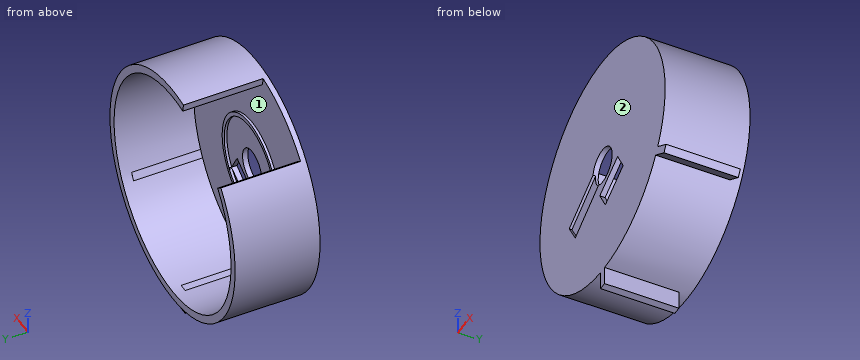
```python
from build123d import *

# Parameters (mm, degrees)
SKETCH1_R                = 45.5
SKETCH1_R_2              = 42.5
BOSS_EXTRUDE1_DEPTH      = 32
SKETCH2_R                = 45.5
BOSS_EXTRUDE2_DEPTH      = 2
SKETCH3_R                = 7
CUT_EXTRUDE1_DEPTH       = 2
SKETCH7_W                = 3
SKETCH7_H                = 10
BOSS_EXTRUDE4_DEPTH      = 26
BOSS_EXTRUDE4_DEPTH_BACK = 2
SKETCH8_R                = 19.890165718
SKETCH8_R_2              = 18.390165718
BOSS_EXTRUDE5_DEPTH      = 1
CUT_EXTRUDE4_DEPTH       = 5.5
CUT_EXTRUDE5_DEPTH       = 58.5
CUT_EXTRUDE6_DEPTH       = 1


with BuildPart() as part:
    # Sketch1 → Boss-Extrude1 (new body)
    with BuildSketch(Plane(origin=(0, 0, 0), x_dir=(1, 0, 0), z_dir=(0, 1, 0))):
        Circle(SKETCH1_R)
        Circle(SKETCH1_R_2, mode=Mode.SUBTRACT)
    extrude(amount=BOSS_EXTRUDE1_DEPTH)

    # Sketch2 → Boss-Extrude2 (add)
    with BuildSketch(Plane.XZ):
        Circle(SKETCH2_R)
    extrude(amount=-BOSS_EXTRUDE2_DEPTH)

    # Sketch3 → Cut-Extrude1 (cut)
    with BuildSketch(Plane(origin=(0, 2, 0), x_dir=(1, 0, 0), z_dir=(0, 1, 0))):
        Circle(SKETCH3_R)
    extrude(amount=-CUT_EXTRUDE1_DEPTH, mode=Mode.SUBTRACT)

    # Sketch7 → Boss-Extrude4 (add, two sides)
    with BuildSketch(Plane(origin=(0, 2, 0), x_dir=(1, 0, 0), z_dir=(0, 1, 0))) as boss_extrude4_sk:
        with Locations((0, 47.473521163)):
            Rectangle(SKETCH7_W, SKETCH7_H)
        Polygon((46.193402353, 24.937722476), (37.533148315, 19.937722476), (36.033148315, 22.535798687), (44.693402353, 27.535798687), align=None)
    extrude(amount=BOSS_EXTRUDE4_DEPTH)
    extrude(boss_extrude4_sk.sketch, amount=-BOSS_EXTRUDE4_DEPTH_BACK)

    # Sketch8 → Boss-Extrude5 (add)
    with BuildSketch(Plane(origin=(0, 2, 0), x_dir=(1, 0, 0), z_dir=(0, 1, 0))):
        Circle(SKETCH8_R)
        Circle(SKETCH8_R_2, mode=Mode.SUBTRACT)
    extrude(amount=BOSS_EXTRUDE5_DEPTH)

    # Sketch10 → Cut-Extrude4 (cut)
    with BuildSketch(Plane.XZ):
        Polygon((2.016687189, -18.494703278), (14.981867268, -10.951222284), (10.958677405, -4.036459575), (-2.006502675, -11.579940569), align=None)
    extrude(amount=-CUT_EXTRUDE4_DEPTH, mode=Mode.SUBTRACT)

    # Sketch11 → Cut-Extrude5 (cut)
    with BuildSketch(Plane(origin=(0, 2, 0), x_dir=(1, 0, 0), z_dir=(0, 1, 0))):
        Polygon((-32.606600292, -26.874098434), (-35.165226496, -28.87311631), (-33.824988888, -37.754161376), (-11.7382848, -48.772412552), (-7.925983096, -44.804338986), (-7.495155029, -41.738838001), (-9.978475631, -35.419229659), (-25.965270809, -26.874098434), align=None)
    extrude(amount=CUT_EXTRUDE5_DEPTH, mode=Mode.SUBTRACT)

    # Sketch12 → Cut-Extrude6 (cut)
    with BuildSketch(Plane.XZ):
        Polygon((-6.912265346, 1.104802147), (-24.20763883, -9.480307189), (-19.814483018, -16.658435267), (-2.519109534, -6.073325931), align=None)
    extrude(amount=-CUT_EXTRUDE6_DEPTH, mode=Mode.SUBTRACT)


solid = part.part
```
Verification items for the finished model (mm, model axes). Face numbers are marked on the shaded views. Give positions to 0.01 mm unless a question says otherwise; leave off trailing zeros. Order: outer loops, then holes, each group sorted by start corner. A loop starts at its lowest first (then second) coordinate and runs counter-clockwise, first axis right, second up. Notation, with made-up numbers: (-18, 27.25) - (26, 27.25) arc R11 cw to (26, 47.25) - close; hole circle Ø10 at (10.25, 16). An arc over 180 degrees is marked (long way). Answer as CSV lines item,"result". Start each with the question number.
Item 1: Material ranges on L1, parallel to Z at x = 0, y = 2.7; L2, parallel to Z at x = 0, y = 13; L3, parallel to Z at x = 0, y = 0.5, recorded low to high.
Item 2: Section check B-B, the plane x = -5. Record the boundary of the cut face in (y, z).
Item 3: Gauge pin test, flat ends, axial feed: pin 1 (5 mm diameter, centred on y = 26.5, z = -11, fed in from +X); pin 2 (22 mm diameter, centred on x = 0, z = 0, fed in from -Y); pin 3 (4 mm diameter, centred on x = -18, y = 16, fed in from -Z); pin 4 (2 mm diameter, centred on y = 17, z = -48, fed in from +X). Record the tip position at first contact, or that the pin passes through.
Item 4: Section check D-D, the plane x = 29. Record the boundary of the cut face in (y, z).
Item 5: Mould release check, pull along X, two halves, no side actions. Record for the marked faces 1 and 2: released by +X, released by -X, zero draft, split by the parting line, or undercut.
Item 6: Section check A-A, the plane y = 25.5. Record the boundary of the cut face in (x, z).
Item 7: Section check C-C, the plane z = 23. Record the boundary of the cut face in (x, y), plus the area to 3 significant figures.
Filled in:
1,L1,"-52.47 to -42.47, -19.89 to -18.39, 18.39 to 19.89, 42.5 to 45.5"
1,L2,"-52.47 to -42.47, 42.5 to 45.5"
1,L3,"-52.47 to -15.03, -10.41 to -7, 7 to 45.5"
2,outline,"(0, -45.22) - (32, -45.22) - (32, -42.2) - (2, -42.2) - (2, -19.25) - (3, -19.25) - (3, -17.7) - (2, -17.7) - (2, -4.9) - (1, -4.9) - (1, -7.59) - (0, -7.59) - close; (0, 4.9) - (2, 4.9) - (2, 17.7) - (3, 17.7) - (3, 19.25) - (2, 19.25) - (2, 42.2) - (32, 42.2) - (32, 45.22) - (0, 45.22) - close"
3,pin 1,"x = 44.7"
3,pin 2,"y = 0"
3,pin 3,"z = -42.59"
3,pin 4,"x = 1.5"
4,outline,"(0, -35.06) - (32, -35.06) - (32, -31.07) - (2, -31.07) - (2, 31.07) - (32, 31.07) - (32, 35.06) - (0, 35.06) - close"
5,face 1,"undercut"
5,face 2,"zero draft"
6,outline,"(-35.17, 28.87) arc R45.5 ccw to (-1.5, -45.48) - (-1.5, -52.47) - (1.5, -52.47) - (1.5, -45.48) arc R45.5 ccw to (38.63, -24.04) - (44.69, -27.54) - (46.19, -24.94) - (40.13, -21.44) arc R45.5 ccw to (-7.93, 44.8) - (-7.51, 41.83) arc R42.5 cw to (37.53, -19.94) - (36.03, -22.54) arc R42.5 cw to (1.5, -42.47) - (-1.5, -42.47) arc R42.5 cw to (-32.8, 27.03) - close"
7,outline,"(-39.26, 0) - (39.26, 0) - (39.26, 32) - (35.74, 32) - (35.74, 2) - (-35.74, 2) - (-35.74, 32) - (-39.26, 32) - close"
7,area,"368 mm^2"
